```python
from build123d import *
from build123d.topology import SkipClean

# Parameters (mm, degrees)
SKETCH1_W           = 76.2
SKETCH1_H           = 101.6
BOSS_EXTRUDE1_DEPTH = 76.2
SKETCH2_RX          = 62.8740047
SKETCH2_RY          = 29.591838086
CUT_EXTRUDE1_DEPTH  = 120.1365603
SHELL1_T            = -3.81
SKETCH4_R           = 2.54
CUT_EXTRUDE2_DEPTH  = 120.13656047
SKETCH5_W           = 139.7
SKETCH5_H           = 127
BOSS_EXTRUDE2_DEPTH = 5.08
CUT_EXTRUDE3_DEPTH  = 122.316579721


with BuildPart() as part:
    # Sketch1 → Boss-Extrude1 (new body)
    with BuildSketch(Plane(origin=(0, 0, 0), x_dir=(1, 0, 0), z_dir=(0, 1, 0))):
        Rectangle(SKETCH1_W, SKETCH1_H)
    extrude(amount=BOSS_EXTRUDE1_DEPTH)

    # Sketch2 → Cut-Extrude1 (cut, through all)
    with SkipClean():  # the faces are left unmerged after this step: merging them gives an invalid solid
        with BuildSketch(Plane.ZY.offset(38.1)):
            with Locations(Location((0, 76.2), (0, 0, -90))):
                Ellipse(SKETCH2_RX, SKETCH2_RY)
        extrude(amount=-CUT_EXTRUDE1_DEPTH, mode=Mode.SUBTRACT)
    add(part.part.scale(1), mode=Mode.REPLACE)  # the faces are merged on a copy

    # Shell1
    shell1_openings = [part.faces().sort_by_distance(p)[0] for p in [
        (0, 76.2, -40.195919043),
        (0, 31.741364916, -20.924589378),
        (0, 31.741364916, 20.924589378),
        (0, 76.2, 40.195919043),
    ]]
    offset(amount=SHELL1_T, openings=shell1_openings, kind=Kind.INTERSECTION)

    # Sketch4 → Cut-Extrude2 (cut, through all)
    with BuildSketch(Plane.ZY.offset(38.1)):
        with Locations((-38.1, 63.5)):
            Circle(SKETCH4_R)
        with Locations((-38.1, 25.4)):
            Circle(SKETCH4_R)
        with Locations(Location((38.1, 25.4, 0), (0, 0, 180))):
            Circle(SKETCH4_R)
        with Locations(Location((38.1, 63.5, 0), (0, 0, 180))):
            Circle(SKETCH4_R)
    extrude(amount=-CUT_EXTRUDE2_DEPTH, mode=Mode.SUBTRACT)

    # Sketch5 → Boss-Extrude2 (add)
    with BuildSketch(Plane.XZ):
        Rectangle(SKETCH5_W, SKETCH5_H)
    extrude(amount=BOSS_EXTRUDE2_DEPTH)

    # Sketch6 → Cut-Extrude3 (cut, through all)
    with BuildSketch(Plane(origin=(0, 0, 0), x_dir=(1, 0, 0), z_dir=(0, 1, 0))):
        with BuildLine():
            Line((-52.07, 44.45), (-52.07, -44.45))
            ThreePointArc((-52.07, -44.45), (-57.15, -49.53), (-62.23, -44.45))
            Line((-62.23, -44.45), (-62.23, 44.45))
            ThreePointArc((-62.23, 44.45), (-57.15, 49.53), (-52.07, 44.45))
        make_face()
        with BuildLine():
            Line((52.07, 44.45), (52.07, -44.45))
            ThreePointArc((52.07, -44.45), (57.15, -49.53), (62.23, -44.45))
            Line((62.23, -44.45), (62.23, 44.45))
            ThreePointArc((62.23, 44.45), (57.15, 49.53), (52.07, 44.45))
        make_face()
    extrude(amount=-CUT_EXTRUDE3_DEPTH, mode=Mode.SUBTRACT)


solid = part.part
```
Work out the finished part from the listing and answer in its coordinate system (mm). A direction names the side the tool comes from. Coordinates: 2 decimals unless noted, no trailing zeros. Loops run counter-clockwise (first coordinate to the right, second up) from the corner with the lowest first, then second, coordinate; pieces in that order, holes last. Notation, with made-up numbers: (63, 38) - (69, 38) arc R9 cw to (69, 42) - close; hole circle Ø9 at (-20.5, -2.5). An arc over 180 degrees is marked (long way). Use a Markdown table: item, result.
Item 1: Find section B-B, the plane x = 57.15. Determine the outline of the cut face in (y, z).
Evaluation:
| item | result |
|---|---|
| outline | (-5.08, -63.5) - (0, -63.5) - (0, -49.53) - (-5.08, -49.53) - close; (-5.08, 49.53) - (0, 49.53) - (0, 63.5) - (-5.08, 63.5) - close |
Item 2: Find section D-D, the plane x = -59. Determine the outline of the cut face in (y, z), and give its area (3 significant figures).
Evaluation:
| item | result |
|---|---|
| outline | (-5.08, -63.5) - (0, -63.5) - (0, -49.18) - (-5.08, -49.18) - close; (-5.08, 49.18) - (0, 49.18) - (0, 63.5) - (-5.08, 63.5) - close |
| area | 145 mm2 |
Item 3: For faces 3 (the cylindrical face through (57.04, -2.5, 49.53)), 4 (the flat face through (-1, 38, 50.8)), 5 (the flat face through (-34.29, 31, 22)), determine the directions among +Z, -Z, +X, -X, +Y, -Y from which every point of the face is accessible in a straight line to the end or side of a thin tool.
Evaluation:
| item | result |
|---|---|
| face 3 | +Y, -Y |
| face 4 | +Z, +X, -X, +Y |
| face 5 | +Y |
Item 4: Given pin 1 Ø20.5 at (x, y) = (4.5, 32.5) entering from -Z; pin 2 Ø10 at (y, z) = (23, 25) entering from +X; pin 3 Ø4 at (y, z) = (25.4, 38.1) entering from +X; pin 4 Ø8 at (y, z) = (25.4, -38.1) entering from -X, each flat-ended and moving along its own axis, determine where each tip first touches the part or whether it passes through.
Evaluation:
| item | result |
|---|---|
| pin 1 | stops at z = -50.8 |
| pin 2 | stops at x = 38.1 |
| pin 3 | passes through |
| pin 4 | stops at x = -38.1 |
Item 5: The mould has two halves that part along X. Classify faces 1 (the flat face through (-52.07, -3, -1)), 2 (the cylindrical face through (36.17, 61.02, -38.65)): +X half, -X half, draft (parallel to the pull), parting line (faces both ways), or undercut.
Evaluation:
| item | result |
|---|---|
| face 1 | undercut |
| face 2 | draft |
Item 6: Find section A-A, the plane z = -32. Determine the outline of the cut face in (x, y), and give its area (3 significant figures).
Evaluation:
| item | result |
|---|---|
| outline | (-69.85, -5.08) - (-62.23, -5.08) - (-62.23, 0) - (-69.85, 0) - close; (-52.07, -5.08) - (52.07, -5.08) - (52.07, 0) - (38.1, 0) - (38.1, 76.2) - (34.29, 76.2) - (34.29, 3.81) - (-34.29, 3.81) - (-34.29, 76.2) - (-38.1, 76.2) - (-38.1, 0) - (-52.07, 0) - close; (62.23, -5.08) - (69.85, -5.08) - (69.85, 0) - (62.23, 0) - close |
| area | 1,450 mm2 |
Item 7: Find section C-C, the plane x = 14. Determine the outline of the cut face in (y, z), and give its area (3 significant figures).
Evaluation:
| item | result |
|---|---|
| outline | (-5.08, -63.5) - (0, -63.5) - (0, -50.8) - (76.2, -50.8) - (76.2, -46.99) - (3.81, -46.99) - (3.81, 46.99) - (76.2, 46.99) - (76.2, 50.8) - (0, 50.8) - (0, 63.5) - (-5.08, 63.5) - close |
| area | 1,580 mm2 |
Item 8: Consider probe 1 along Y at (x, z) = (36.5, -38.1); probe 2 along X at (y, z) = (52, -31); probe 3 along Z at (x, y) = (13, 70). Determine where each line is inside the solid, lowest interval first. Write a range as from..to.
Evaluation:
| item | result |
|---|---|
| probe 1 | y = -5.08..22.86, 27.94..60.96, 66.04..76.2 |
| probe 2 | x = -38.1..-34.29, 34.29..38.1 |
| probe 3 | z = -50.8..-46.99, 46.99..50.8 |
